Check sheet for the modelled part. Datum: model origin and axes. Units: mm. Face numbers are marked on the shaded views. A direction names the side the tool comes from. Coordinates: 2 decimals unless noted, no trailing zeros. Loops run counter-clockwise (first coordinate to the right, second up) from the corner with the lowest first, then second, coordinate; pieces in that order, holes last.
```python
from build123d import *

# Parameters (mm, degrees)
ESQUISSE1_W             = 70
ESQUISSE1_H             = 25
BOSS_EXTRU_1_DEPTH      = 21
ESQUISSE2_W             = 68
ESQUISSE2_H             = 22
ENL_V_MAT_EXTRU_1_DEPTH = 19
ESQUISSE3_W             = 18
ESQUISSE3_H             = 22
ESQUISSE3_W_2           = 1
ESQUISSE3_H_2           = 6
BOSS_EXTRU_2_DEPTH      = 6
ESQUISSE4_W             = 8
ESQUISSE4_H             = 3
ESQUISSE4_W_2           = 4
ESQUISSE4_H_2           = 2
ESQUISSE4_W_3           = 6
ESQUISSE4_H_3           = 8
ENL_V_MAT_EXTRU_2_DEPTH = 4
CHANFREIN1_SIZE         = 2


with BuildPart() as part:
    # Esquisse1 → Boss.-Extru.1 (new body)
    with BuildSketch(Plane(origin=(0, 0, 0), x_dir=(1, 0, 0), z_dir=(0, 1, 0))):
        with Locations((35, 12.5)):
            Rectangle(ESQUISSE1_W, ESQUISSE1_H)
    extrude(amount=BOSS_EXTRU_1_DEPTH)

    # Esquisse2 → Enlèv. mat.-Extru.1 (cut)
    with BuildSketch(Plane(origin=(0, 21, 0), x_dir=(1, 0, 0), z_dir=(0, 1, 0))):
        with Locations((35, 12.5)):
            Rectangle(ESQUISSE2_W, ESQUISSE2_H)
    extrude(amount=-ENL_V_MAT_EXTRU_1_DEPTH, mode=Mode.SUBTRACT)

    # Esquisse3 → Boss.-Extru.2 (add)
    with BuildSketch(Plane(origin=(0, 2, 0), x_dir=(1, 0, 0), z_dir=(0, 1, 0))):
        with Locations((60, 12.5)):
            Rectangle(ESQUISSE3_W, ESQUISSE3_H)
        with Locations((23.881932789, 20.5)):
            Rectangle(ESQUISSE3_W_2, ESQUISSE3_H_2)
        with Locations((39.638895705, 20.5)):
            Rectangle(ESQUISSE3_W_2, ESQUISSE3_H_2)
        with Locations((22.463097558, 4.5)):
            Rectangle(ESQUISSE3_W_2, ESQUISSE3_H_2)
        with Locations((39.638895705, 4.5)):
            Rectangle(ESQUISSE3_W_2, ESQUISSE3_H_2)
    extrude(amount=BOSS_EXTRU_2_DEPTH)

    # Esquisse4 → Enlèv. mat.-Extru.2 (cut)
    with BuildSketch(Plane(origin=(70, 0, 0), x_dir=(0, 0, -1), z_dir=(1, 0, 0))):
        with Locations((6.5, 4.5)):
            Rectangle(ESQUISSE4_W, ESQUISSE4_H)
        with Locations((14.742986582, 4)):
            Rectangle(ESQUISSE4_W_2, ESQUISSE4_H_2)
        with Locations((22, 4)):
            Rectangle(ESQUISSE4_W_3, ESQUISSE4_H_3)
    extrude(amount=-ENL_V_MAT_EXTRU_2_DEPTH, mode=Mode.SUBTRACT)

    # Chanfrein1
    chanfrein1_edges = [part.edges().sort_by_distance(p)[0] for p in [
        (33, 0, -25),
        (70, 0, -9.5),
        (35, 0, 0),
        (0, 0, -12.5),
    ]]
    chamfer(chanfrein1_edges, length=CHANFREIN1_SIZE)


solid = part.part
```
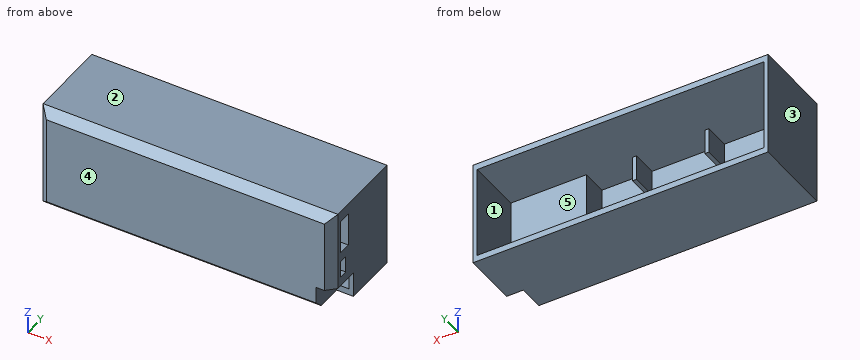
1) Section check D-D on x = 52.5. Enter the section's corners in (y, z).
Answer sheet:
outline: (0, -23) - (2, -25) - (21, -25) - (21, -23.5) - (8, -23.5) - (8, -1.5) - (21, -1.5) - (21, 0) - (2, 0) - (0, -2) - close
2) Section check B-B on x = 42.5. Enter the section's corners in (y, z), plus the area to 3 significant figures.
Answer sheet:
outline: (0, -23) - (2, -25) - (21, -25) - (21, -23.5) - (2, -23.5) - (2, -1.5) - (21, -1.5) - (21, 0) - (2, 0) - (0, -2) - close
area: 103 mm2
3) Section check C-C on z = -8.5. Enter the section's corners in (x, y).
Answer sheet:
outline: (0, 2) - (2, 0) - (68, 0) - (70, 2) - (70, 3) - (66, 3) - (66, 6) - (70, 6) - (70, 21) - (69, 21) - (69, 8) - (51, 8) - (51, 2) - (1, 2) - (1, 21) - (0, 21) - close
4) Section check A-A on y = 12.25. Enter the section's corners in (x, z).
Answer sheet:
outline: (0, -25) - (70, -25) - (70, 0) - (0, 0) - close; hole (1, -23.5) - (69, -23.5) - (69, -1.5) - (1, -1.5) - close
5) Mould release check, pull along X, two halves, no side actions. Record for the marked faces 3, 4 and 5: +X half, -X half, draft (parallel to the pull), parting line (faces both ways), or undercut.
Answer sheet:
face 3: -X half
face 4: draft
face 5: undercut
6) Scan lines: line 1 (X direction, y = 6, z = -22); line 2 (X direction, y = 20.25, z = -2.5); line 3 (Z direction, x = 29, y = 7). Record each from-to range of solid material in increasing order.
Answer sheet:
line 1: x = 0 to 1, 23.38 to 24.38, 39.14 to 40.14, 51 to 66
line 2: x = 0 to 1, 69 to 70
line 3: z = -25 to -23.5, -1.5 to 0
7) Depth check by flat-ended pin: pin 1 (6 mm diameter, centred on y = 14, z = -8, fed in from -X); pin 2 (4 mm diameter, centred on x = 34, z = -11.5, fed in from +Y); pin 3 (1 mm diameter, centred on x = 67, y = 4, fed in from -Z); pin 4 (2 mm diameter, centred on x = 52, z = -6.5, fed in from +Y). Enter the tip coordinate at first touch or a pass-through.
Answer sheet:
pin 1: stops at x = 0
pin 2: stops at y = 2
pin 3: stops at z = -19
pin 4: stops at y = 8
8) Set-up check for the marked faces 1 and 2: record each of +Z, -Z, +X, -X, +Y, -Y from which the full face is reachable in a straight line by a thin tool's end or side.
Answer sheet:
face 1: +Y
face 2: +Z, +X, -X, +Y, -Y
